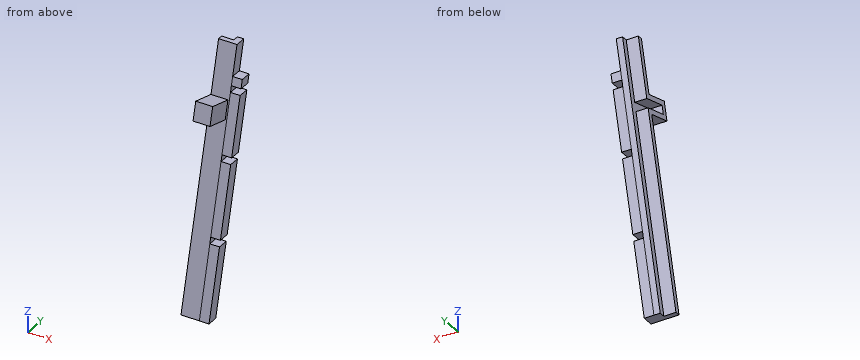
```python
from build123d import *

# Parameters (mm, degrees)
SIDE_COMB_DEPTH           = 4
SIDE_COMB_2_DEPTH         = 4
SIDE_COMB_3_DEPTH         = 4
SIDE_COMB_4_DEPTH         = 4
SIDE_SPACER_DEPTH         = 2.6
NARROW_SUPPORT_DEPTH      = 5
SKETCH7_W                 = 5
SKETCH7_H                 = 3.5
GAP_FOR_SUPPORT_BAR_DEPTH = 2
SUPPORT_BAR_SIDES_DEPTH   = 8.5
SKETCH8_W                 = 7
SKETCH8_H                 = 7.5
SUPPORT_BAR_BOTTOM_DEPTH  = 2


with BuildPart() as part:
    # Sketch1 → Side comb (new body)
    with BuildSketch(Plane(origin=(0, 0, 0), x_dir=(0, 0, -1), z_dir=(1, 0, 0))):
        Polygon((3.396035042, -0.846726635), (0, 0), (0, -4.5), (3.396035042, -5.346726635), align=None)
    extrude(amount=SIDE_COMB_DEPTH)



with BuildPart() as body_2:
    # Sketch1 → Side comb 2 (new body)
    with BuildSketch(Plane(origin=(0, 0, 0), x_dir=(0, 0, -1), z_dir=(1, 0, 0))):
        Polygon((28.623723925, -7.13669592), (5.821774358, -1.451531374), (5.821774358, -5.951531374), (28.623723925, -11.63669592), align=None)
    extrude(amount=SIDE_COMB_2_DEPTH)


with BuildPart() as body_3:
    # Sketch1 → Side comb 3 (new body)
    with BuildSketch(Plane(origin=(0, 0, 0), x_dir=(0, 0, -1), z_dir=(1, 0, 0))):
        Polygon((58.70289144, -14.636274684), (31.049463241, -7.741500659), (31.049463241, -12.241500659), (58.70289144, -19.136274684), align=None)
    extrude(amount=SIDE_COMB_3_DEPTH)


with BuildPart() as body_4:
    # Sketch1 → Side comb 4 (new body)
    with BuildSketch(Plane(origin=(0, 0, 0), x_dir=(0, 0, -1), z_dir=(1, 0, 0))):
        Polygon((89.267206817, -22.256814395), (61.128630755, -15.241079423), (61.128630755, -19.741079423), (89.267206817, -26.756814395), align=None)
    extrude(amount=SIDE_COMB_4_DEPTH)


with BuildPart() as part_1:
    add(part.part)

    add(body_2.part)  # Side spacer merges body 2

    add(body_3.part)  # Side spacer merges body 3

    add(body_4.part)  # Side spacer merges body 4
    # Sketch2 → Side spacer (add)
    with BuildSketch(Plane.ZY):
        Polygon((-89.267206817, -22.256814395), (-89.267206817, -26.756814395), (11.643548715, -1.596937253), (11.643548715, 2.903062747), align=None)
    extrude(amount=SIDE_SPACER_DEPTH)

    # Sketch3 → Narrow support (add)
    with BuildSketch(Plane.ZY.offset(2.6)):
        Polygon((-89.267206817, -24.695587136), (11.643548715, 0.464290006), (11.643548715, -1.596937253), (-89.267206817, -26.756814395), align=None)
    extrude(amount=NARROW_SUPPORT_DEPTH)

    # Sketch7 → Gap for support bar (cut)
    with BuildSketch(Plane(origin=(0, -4.236632084, 1.056311016), x_dir=(1, 0, 0), z_dir=(0, -0.970295726, 0.241921896))):
        with Locations((-5.1, -13.839992525)):
            Rectangle(SKETCH7_W, SKETCH7_H)
    extrude(amount=-GAP_FOR_SUPPORT_BAR_DEPTH, mode=Mode.SUBTRACT)

    # Sketch6 → Support bar sides (add)
    with BuildSketch(Plane(origin=(0, -4.236632084, 1.056311016), x_dir=(1, 0, 0), z_dir=(0, -0.970295726, 0.241921896))):
        Polygon((-2.6, -12.089992525), (-7.6, -12.089992525), (-7.6, -10.089992525), (-0.6, -10.089992525), (-0.6, -17.589992525), (-7.6, -17.589992525), (-7.6, -15.589992525), (-2.6, -15.589992525), align=None)
    extrude(amount=SUPPORT_BAR_SIDES_DEPTH)

    # Sketch8 → Support bar bottom (add)
    with BuildSketch(Plane(origin=(0, -12.484145757, 3.112647129), x_dir=(1, 0, 0), z_dir=(0, -0.970295726, 0.241921896))):
        with Locations((-4.1, -13.839992525)):
            Rectangle(SKETCH8_W, SKETCH8_H)
    extrude(amount=SUPPORT_BAR_BOTTOM_DEPTH)


solid = part_1.part
```
Verification items for the finished model (mm, model axes). Give positions to 0.01 mm unless a question says otherwise; leave off trailing zeros. Order: outer loops, then holes, each group sorted by start corner. A loop starts at its lowest first (then second) coordinate and runs counter-clockwise, first axis right, second up. Notation, with made-up numbers: (78.5, 3) - (125.5, 3) arc R15 ccw to (125.5, 14) - close; hole circle Ø2 at (44.25, -39). An arc over 180 degrees is marked (long way). Answer as CSV lines item,"result". Start each with the question number.
Item 1: Gauge pin test, flat ends, axial feed: pin 1 (1.2 mm diameter, centred on x = 1.5, y = -1.5, fed in from +Z); pin 2 (1.2 mm diameter, centred on y = -2, z = -5, fed in from +X); pin 3 (8 mm diameter, centred on y = -11.5, z = -10, fed in from +X). Record the tip position at first contact, or that the pin passes through.
Item 2: Section check A-A, the plane x = 1. Record the boundary of the cut face in (y, z), plus the area to 3 significant figures.
Item 3: Section check B-B, the plane y = -2.5. Record the boundary of the cut face in (x, z).
Item 4: Section check D-D, the plane z = -80. Record the boundary of the cut face in (x, y).
Item 5: Section check C-C, the plane x = -5.5. Record the boundary of the cut face in (y, z).
Item 6: Material ranges on L1, parallel to X at y = -17, z = -7; L2, parallel to X at y = -4.5, z = -12; L3, parallel to Y at x = -4.75, z = -6, recorded low to high.
Filled in:
1,pin 1,"z = 0"
1,pin 2,"x = 0"
1,pin 3,"x = -0.6"
2,outline,"(-26.76, -89.27) - (-22.26, -89.27) - (-15.24, -61.13) - (-19.74, -61.13) - close; (-19.14, -58.7) - (-14.64, -58.7) - (-7.74, -31.05) - (-12.24, -31.05) - close; (-11.64, -28.62) - (-7.14, -28.62) - (-1.45, -5.82) - (-5.95, -5.82) - close; (-5.35, -3.4) - (-0.85, -3.4) - (0, 0) - (-4.5, 0) - close"
2,area,"369 mm^2"
3,outline,"(-7.6, -0.25) - (-2.6, -0.25) - (-2.6, -10.03) - (4, -10.03) - (4, -5.82) - (0, -5.82) - (0, -3.4) - (4, -3.4) - (4, 0) - (0, 0) - (0, 8.02) - (-7.6, 8.02) - close"
4,outline,"(-7.6, -24.45) - (4, -24.45) - (4, -19.95) - (-2.6, -19.95) - (-2.6, -22.39) - (-7.6, -22.39) - close"
5,outline,"(-26.76, -89.27) - (-24.7, -89.27) - (-6.07, -14.55) - (-16.26, -12.01) - (-15.41, -8.62) - (-5.22, -11.16) - (0.46, 11.64) - (-1.6, 11.64) - (-6.68, -8.73) - (-16.87, -6.19) - (-18.68, -13.47) - (-8.49, -16.01) - close"
6,L1,"-7.6 to -0.6"
6,L2,"-2.6 to 4"
6,L3,"-6 to -3.93"
